CAD build for the part. Positions are in the model's coordinates, mm. A direction names the side the tool comes from. Coordinates: 2 decimals unless noted, no trailing zeros. Loops run counter-clockwise (first coordinate to the right, second up) from the corner with the lowest first, then second, coordinate; pieces in that order, holes last.
1) Saw through at A-A, the plane y = -18. Write the cut outline in (x, z), and give its area (3 significant figures).
2) Pin check, flat tips, straight feed: pin 1 Ø3 at (x, y) = (7, 43.5) entering from +Z; pin 2 Ø1.6 at (x, y) = (1.5, -12.5) entering from -Z; pin 3 Ø16 at (x, z) = (15.5, -136.5) entering from +Y. Stop position of each tip, or through.
3) Two-plate mould, pull along Y, no slides. Class faces 6 (the flat face through (5, -60, 1)), 7 (the flat face through (26, 10, 150)), 8 (the cylindrical face through (5.944, -35.743, 9.229)), 9 (the cylindrical face through (4.93, 28.85, -63.01)): +Y half, -Y half, draft (parallel to the pull), parting line (faces both ways), or undercut.
4) Wall check: line 1 along Y through (x, z) = (4.5, -36.77); line 2 along Z through (x, y) = (15.5, -17.5); line 3 along Y through (x, z) = (6, -36). Give the ranges that are in metal, low to high.
5) Saw through at D-D, the plane z = 0. Write the cut outline in (x, y).
6) Saw through at C-C, the plane z = 170. Write the cut outline in (x, y).
7) Which spindle directions (+Z, -Z, +X, -X, +Y, -Y) get a long thin tool onto all of the face, cutting with end or side? Do faces 1 (the flat face through (5, -43, 60)), 2 (the flat face through (16, 0, -190)), 3 (the flat face through (5, -43, -60)), 4 (the cylindrical face through (-13.804, -4.788, -154.795)), 5 (the flat face through (10, 14, -1)). Say none if no direction does.
8) Saw through at B-B, the plane x = 43.5. Write the cut outline in (y, z), and give its area (3 significant figures).
```python
from build123d import *

# Parameters (mm, degrees)
SKETCH_1_W                  = 52
SKETCH_1_H                  = 380
EXTRUDE_1_DEPTH             = 52
SKETCH_2_W                  = 42
SKETCH_2_H                  = 285
CUT_EXTRUDE_1_DEPTH         = 204.735122156
SKETCH_3_W                  = 95
SKETCH_3_H                  = 52
EXTRUDE_2_DEPTH             = 22
SKETCH_4_W                  = 10
SKETCH_4_H                  = 120
EXTRUDE_3_DEPTH             = 34
SKETCH_5_W                  = 10
SKETCH_5_H                  = 120
EXTRUDE_4_DEPTH             = 34
SKETCH_6_W                  = 40
SKETCH_6_H                  = 32
CUT_EXTRUDE_2_DEPTH         = 206.922315449
SKETCH_7_W                  = 91
SKETCH_7_H                  = 91
CUT_EXTRUDE_3_DEPTH         = 2
SKETCH_8_W                  = 28
SKETCH_8_H                  = 12.5
SKETCH_9_W                  = 26
SKETCH_9_H                  = 12.5
HOLE_WIZARD_13_0_13_1_D     = 13
HOLE_WIZARD_13_0_13_1_DEPTH = 86
HOLE_WIZARD_M39_1_D         = 40
HOLE_WIZARD_M39_1_DEPTH     = 38
HOLE_WIZARD_6_0_6_1_D       = 6
HOLE_WIZARD_6_0_6_1_DEPTH   = 38
FILLET_1_R                  = 5
FILLET_2_R                  = 10


with BuildPart() as part:
    # 草图1 → 凸台-拉伸1 (new body)
    with BuildSketch(Plane(origin=(0, 26, 0), x_dir=(1, 0, 0), z_dir=(0, 1, 0))):
        with Locations((26, 0)):
            Rectangle(SKETCH_1_W, SKETCH_1_H)
    extrude(amount=-EXTRUDE_1_DEPTH)

    # 草图2 → 切除-拉伸1 (cut, through all)
    with BuildSketch(Plane(origin=(0, 26, 0), x_dir=(-1, 0, 0), z_dir=(0, 1, 0))):
        with Locations((-31, -47.5)):
            Rectangle(SKETCH_2_W, SKETCH_2_H)
    extrude(amount=-CUT_EXTRUDE_1_DEPTH, mode=Mode.SUBTRACT)

    # 草图3 → 凸台-拉伸2 (add)
    with BuildSketch(Plane(origin=(10, 0, 0), x_dir=(0, 0, -1), z_dir=(1, 0, 0))):
        with Locations((142.5, 0)):
            Rectangle(SKETCH_3_W, SKETCH_3_H)
    extrude(amount=EXTRUDE_2_DEPTH)

    # 草图4 → 凸台-拉伸3 (add)
    with BuildSketch(Plane(origin=(0, 26, 0), x_dir=(-1, 0, 0), z_dir=(0, 1, 0))):
        with Locations((-5, 0)):
            Rectangle(SKETCH_4_W, SKETCH_4_H)
    extrude(amount=EXTRUDE_3_DEPTH)

    # 草图5 → 凸台-拉伸4 (add)
    with BuildSketch(Plane.XZ.offset(26)):
        with Locations((5, 0)):
            Rectangle(SKETCH_5_W, SKETCH_5_H)
    extrude(amount=EXTRUDE_4_DEPTH)

    # 草图6 → 切除-拉伸2 (cut, through all)
    with BuildSketch(Plane.ZY):
        with Locations((170, 10)):
            Rectangle(SKETCH_6_W, SKETCH_6_H)
    extrude(amount=-CUT_EXTRUDE_2_DEPTH, mode=Mode.SUBTRACT)

    # 草图7 → 切除-拉伸3 (cut)
    with BuildSketch(Plane.ZY):
        Rectangle(SKETCH_7_W, SKETCH_7_H)
    extrude(amount=-CUT_EXTRUDE_3_DEPTH, mode=Mode.SUBTRACT)

    # 草图8 → 旋转1 (revolve)
    with BuildSketch(Plane.XY.offset(-143.248009954), mode=Mode.PRIVATE) as revolve_1_sk:
        with Locations((-14, 6.25)):
            Rectangle(SKETCH_8_W, SKETCH_8_H)
    revolve(revolve_1_sk.sketch.rotate(Axis((-28, 0, -143.248009954), (1, 0, 0)), 270), axis=Axis((-28, 0, -143.248009954), (1, 0, 0)))

    # 草图9 → 旋转2 (revolve)
    with BuildSketch(Plane.XY.offset(-143.248009954), mode=Mode.PRIVATE) as revolve_2_sk:
        with Locations((45, 6.25)):
            Rectangle(SKETCH_9_W, SKETCH_9_H)
    revolve(revolve_2_sk.sketch.rotate(Axis((32, 0, -143.248009954), (1, 0, 0)), 270), axis=Axis((32, 0, -143.248009954), (1, 0, 0)))

    # Ø13.0 (13) 直径孔1
    with Locations(Plane(origin=(0, -26, 0), x_dir=(-1, 0, 0), z_dir=(0, -1, 0))):
        with Locations((-32, -170)):
            Hole(HOLE_WIZARD_13_0_13_1_D / 2, depth=HOLE_WIZARD_13_0_13_1_DEPTH)

    # M39 螺旋的螺纹孔钻头1
    with Locations(Plane(origin=(10, 0, 0), x_dir=(0, 0, -1), z_dir=(1, 0, 0))):
        with Locations((0, -18)):
            Hole(HOLE_WIZARD_M39_1_D / 2, depth=HOLE_WIZARD_M39_1_DEPTH)

    # Ø6.0 (6) 直径孔1
    with Locations(Plane(origin=(10, 0, 0), x_dir=(0, 0, -1), z_dir=(1, 0, 0))):
        with Locations((36.77, 36.77), (36.77, -36.77), (-36.77, -36.77), (-36.77, 36.77)):
            Hole(HOLE_WIZARD_6_0_6_1_D / 2, depth=HOLE_WIZARD_6_0_6_1_DEPTH)

    # 圆角1
    fillet_1_edges = [part.edges().sort_by_distance(p)[0] for p in [
        (52, 0, 95),
        (10, 0, 95),
        (10, 0, -95),
        (32, 0, -190),
        (32, 0, -95),
        (52, 10, 150),
        (0, 10, 150),
        (0, -16, 190),
        (0, 0, -190),
        (52, -16, 190),
        (1, 45.5, -45.5),
        (1, 45.5, 45.5),
        (1, -45.5, 45.5),
        (1, -45.5, -45.5),
    ]]
    fillet(fillet_1_edges, radius=FILLET_1_R)

    # 圆角2
    fillet_2_edges = [part.edges().sort_by_distance(p)[0] for p in [
        (5, 26, 60),
        (5, 26, -60),
        (5, 60, 60),
        (5, 60, -60),
        (5, -26, -60),
        (5, -26, 60),
        (5, -60, -60),
        (5, -60, 60),
    ]]
    fillet(fillet_2_edges, radius=FILLET_2_R)


solid = part.part
```
Data:
1. outline: (0, -185) arc R5 ccw to (5, -190) - (27, -190) arc R5 ccw to (32, -185) - (32, -100) arc R5 ccw to (27, -95) - (15, -95) arc R5 cw to (10, -90) - (10, -20) - (2, -20) - (2, -45.5) - (0, -45.5) - close; (0, 45.5) - (2, 45.5) - (2, 20) - (10, 20) - (10, 90) arc R5 cw to (15, 95) - (47, 95) arc R5 ccw to (52, 100) - (52, 185) arc R5 ccw to (47, 190) - (5, 190) arc R5 ccw to (0, 185) - close; hole circle Ø13 at (32, 170)
1. area: 9,220 mm2
2. pin 1: stops at z = 60
2. pin 2: stops at z = -189.21
2. pin 3: stops at y = 26
3. face 6: -Y half
3. face 7: draft
3. face 8: undercut
3. face 9: +Y half
4. line 1: y = -60 to -39.77, -33.77 to 33.77, 39.77 to 60
4. line 2: z = -190 to -95, 95 to 190
4. line 3: y = -60 to -39.67, -33.87 to 33.87, 39.67 to 60
5. outline: (0, -60) - (10, -60) - (10, -38) - (2, -38) - (2, -45.5) - (0, -45.5) - close; (0, 45.5) - (2, 45.5) - (2, 2) - (10, 2) - (10, 60) - (0, 60) - close
6. outline: (0, -26) - (25.5, -26) - (25.5, -6) - (0, -6) - close; (38.5, -26) - (52, -26) - (52, -6) - (38.5, -6) - close
7. face 1: +Z, +X, -X, -Y
7. face 2: -Z, +X, -X, +Y, -Y
7. face 3: -Z, +X, -X, -Y
7. face 4: -X
7. face 5: +X, +Y, -Y
8. outline: (-26, 95) - (26, 95) - (26, 150) - (-6, 150) - (-6, 190) - (-26, 190) - close; circle Ø25 at (0, -143.25)
8. area: 4,150 mm2
